Source: CAD feature listing. Evaluate the final solid. Frame: model axes, mm. A direction names the side the tool comes from. Round coordinates to 2 decimals unless told otherwise and drop trailing zeros. Write each loop counter-clockwise with the first axis right and the second up, starting at its lowest first coordinate (ties: lowest second). Pieces come first, ordered by that corner, then holes. Notation, with made-up numbers: (60, -25) - (69, -25) arc R10 cw to (69, -20) - close; hole circle Ø5 at (27, 76.5). An arc over 180 degrees is marked (long way). Write item = value, one per line. Start each with the question number.
```python
from build123d import *

# Parameters (mm, degrees)
BOSS_EXTRUDE2_DEPTH   = 3
BOSS_EXTRUDE2_2_DEPTH = 3
BOSS_EXTRUDE2_3_DEPTH = 3
BOSS_EXTRUDE2_4_DEPTH = 3
BOSS_EXTRUDE2_5_DEPTH = 3
SKETCH1_3_R           = 1.495691171
SKETCH1_3_R_2         = 1.676523608
BOSS_EXTRUDE3_DEPTH   = 2.5
SKETCH4_R             = 2
CUT_EXTRUDE5_DEPTH    = 69.0734897
CHAMFER1_SIZE         = 0.05


with BuildPart() as part:
    # Sketch1 → Boss-Extrude2 (new, symmetric)
    with BuildSketch(Plane.XY):
        with BuildLine():
            Line((-27.5, 20), (27.5, 20))
            ThreePointArc((27.5, 20), (31.035533906, 18.535533906), (32.5, 15))
            Line((32.5, 15), (32.5, -15))
            ThreePointArc((32.5, -15), (31.035533906, -18.535533906), (27.5, -20))
            Line((27.5, -20), (-27.5, -20))
            ThreePointArc((-27.5, -20), (-31.035533906, -18.535533906), (-32.5, -15))
            Line((-32.5, -15), (-32.5, 15))
            ThreePointArc((-32.5, 15), (-31.035533906, 18.535533906), (-27.5, 20))
        make_face()
        with BuildLine():
            Line((-31.5, 15), (-31.5, -15))
            ThreePointArc((-31.5, -15), (-30.328427125, -17.828427125), (-27.5, -19))
            Line((-27.5, -19), (27.5, -19))
            ThreePointArc((27.5, -19), (30.328427125, -17.828427125), (31.5, -15))
            Line((31.5, -15), (31.5, 15))
            ThreePointArc((31.5, 15), (30.328427125, 17.828427125), (27.5, 19))
            Line((27.5, 19), (-27.5, 19))
            ThreePointArc((-27.5, 19), (-30.328427125, 17.828427125), (-31.5, 15))
        make_face(mode=Mode.SUBTRACT)
    extrude(amount=BOSS_EXTRUDE2_DEPTH, both=True)



with BuildPart() as body_2:
    # Sketch1 → Boss-Extrude2 2 (new, symmetric)
    with BuildSketch(Plane.XY):
        with BuildLine():
            Line((-26.014041324, 17.60613254), (-13.852089473, 10.671658719))
            ThreePointArc((-13.852089473, 10.671658719), (-12.731915609, 6.579567504), (-16.824006824, 5.45939364))
            Line((-16.824006824, 5.45939364), (-28.985958676, 12.39386746))
            ThreePointArc((-28.985958676, 12.39386746), (-30.10613254, 16.485958676), (-26.014041324, 17.60613254))
        make_face()
        with BuildLine():
            Line((-26.261701104, 17.171777116), (-14.099749252, 10.237303296))
            ThreePointArc((-14.099749252, 10.237303296), (-13.166271032, 6.827227283), (-16.576347045, 5.893749063))
            Line((-16.576347045, 5.893749063), (-28.738298896, 12.828222884))
            ThreePointArc((-28.738298896, 12.828222884), (-29.671777116, 16.238298896), (-26.261701104, 17.171777116))
        make_face(mode=Mode.SUBTRACT)
    extrude(amount=BOSS_EXTRUDE2_2_DEPTH, both=True)


with BuildPart() as body_3:
    # Sketch1 → Boss-Extrude2 3 (new, symmetric)
    with BuildSketch(Plane.XY):
        with BuildLine():
            Line((26.014041324, 17.60613254), (13.852089473, 10.671658719))
            ThreePointArc((13.852089473, 10.671658719), (12.731915609, 6.579567504), (16.824006824, 5.45939364))
            Line((16.824006824, 5.45939364), (28.985958676, 12.39386746))
            ThreePointArc((28.985958676, 12.39386746), (30.10613254, 16.485958676), (26.014041324, 17.60613254))
        make_face()
        with BuildLine():
            Line((26.261701104, 17.171777116), (14.099749252, 10.237303296))
            ThreePointArc((14.099749252, 10.237303296), (13.166271032, 6.827227283), (16.576347045, 5.893749063))
            Line((16.576347045, 5.893749063), (28.738298896, 12.828222884))
            ThreePointArc((28.738298896, 12.828222884), (29.671777116, 16.238298896), (26.261701104, 17.171777116))
        make_face(mode=Mode.SUBTRACT)
    extrude(amount=BOSS_EXTRUDE2_3_DEPTH, both=True)


with BuildPart() as body_4:
    # Sketch1 → Boss-Extrude2 4 (new, symmetric)
    with BuildSketch(Plane.XY):
        with BuildLine():
            Line((26.014041324, -17.60613254), (13.852089473, -10.671658719))
            ThreePointArc((13.852089473, -10.671658719), (12.731915609, -6.579567504), (16.824006824, -5.45939364))
            Line((16.824006824, -5.45939364), (28.985958676, -12.39386746))
            ThreePointArc((28.985958676, -12.39386746), (30.10613254, -16.485958676), (26.014041324, -17.60613254))
        make_face()
        with BuildLine():
            Line((26.261701104, -17.171777116), (14.099749252, -10.237303296))
            ThreePointArc((14.099749252, -10.237303296), (13.166271032, -6.827227283), (16.576347045, -5.893749063))
            Line((16.576347045, -5.893749063), (28.738298896, -12.828222884))
            ThreePointArc((28.738298896, -12.828222884), (29.671777116, -16.238298896), (26.261701104, -17.171777116))
        make_face(mode=Mode.SUBTRACT)
    extrude(amount=BOSS_EXTRUDE2_4_DEPTH, both=True)


with BuildPart() as body_5:
    # Sketch1 → Boss-Extrude2 5 (new, symmetric)
    with BuildSketch(Plane.XY):
        with BuildLine():
            Line((-26.014041324, -17.60613254), (-13.852089473, -10.671658719))
            ThreePointArc((-13.852089473, -10.671658719), (-12.731915609, -6.579567504), (-16.824006824, -5.45939364))
            Line((-16.824006824, -5.45939364), (-28.985958676, -12.39386746))
            ThreePointArc((-28.985958676, -12.39386746), (-30.10613254, -16.485958676), (-26.014041324, -17.60613254))
        make_face()
        with BuildLine():
            Line((-26.261701104, -17.171777116), (-14.099749252, -10.237303296))
            ThreePointArc((-14.099749252, -10.237303296), (-13.166271032, -6.827227283), (-16.576347045, -5.893749063))
            Line((-16.576347045, -5.893749063), (-28.738298896, -12.828222884))
            ThreePointArc((-28.738298896, -12.828222884), (-29.671777116, -16.238298896), (-26.261701104, -17.171777116))
        make_face(mode=Mode.SUBTRACT)
    extrude(amount=BOSS_EXTRUDE2_5_DEPTH, both=True)


with BuildPart() as part_1:
    add(part.part)

    add(body_2.part)  # Boss-Extrude3 merges body 2

    add(body_3.part)  # Boss-Extrude3 merges body 3

    add(body_4.part)  # Boss-Extrude3 merges body 4

    add(body_5.part)  # Boss-Extrude3 merges body 5
    # Sketch1_3 → Boss-Extrude3 (add, symmetric)
    with BuildSketch(Plane.XY):
        with BuildLine():
            ThreePointArc((-27.5, 19), (-30.328427125, 17.828427125), (-31.5, 15))
            Line((-31.5, 15), (-31.5, -15))
            ThreePointArc((-31.5, -15), (-30.328427125, -17.828427125), (-27.5, -19))
            Line((-27.5, -19), (27.5, -19))
            ThreePointArc((27.5, -19), (30.328427125, -17.828427125), (31.5, -15))
            Line((31.5, -15), (31.5, 15))
            ThreePointArc((31.5, 15), (30.328427125, 17.828427125), (27.5, 19))
            Line((27.5, 19), (-27.5, 19))
        make_face()
        with BuildLine():
            Line((-13.852089473, -10.671658719), (-26.014041324, -17.60613254))
            ThreePointArc((-26.014041324, -17.60613254), (-30.10613254, -16.485958676), (-28.985958676, -12.39386746))
            Line((-28.985958676, -12.39386746), (-16.824006824, -5.45939364))
            ThreePointArc((-16.824006824, -5.45939364), (-12.731915609, -6.579567504), (-13.852089473, -10.671658719))
        make_face(mode=Mode.SUBTRACT)
        with BuildLine():
            ThreePointArc((0, -17.607662989), (-6.244508299, -12.814840409), (-8.638223432, -5.315829804))
            Line((-8.638223432, -5.315829804), (-7.540721224, -4.64044383))
            ThreePointArc((-7.540721224, -4.64044383), (-4.327491025, -12.392789568), (3.48180896, -15.465011321))
            Line((3.48180896, -15.465011321), (0, -17.607662989))
        make_face(mode=Mode.SUBTRACT)
        with Locations((4.527145443, -11.53276309)):
            Circle(SKETCH1_3_R, mode=Mode.SUBTRACT)
        with BuildLine():
            ThreePointArc((28.985958676, -12.39386746), (30.10613254, -16.485958676), (26.014041324, -17.60613254))
            Line((26.014041324, -17.60613254), (13.852089473, -10.671658719))
            ThreePointArc((13.852089473, -10.671658719), (12.731915609, -6.579567504), (16.824006824, -5.45939364))
            Line((16.824006824, -5.45939364), (28.985958676, -12.39386746))
        make_face(mode=Mode.SUBTRACT)
        with Locations((1.848455798, -6.957616723)):
            Circle(SKETCH1_3_R_2, mode=Mode.SUBTRACT)
        with BuildLine():
            ThreePointArc((-28.985958676, 12.39386746), (-30.10613254, 16.485958676), (-26.014041324, 17.60613254))
            Line((-26.014041324, 17.60613254), (-13.852089473, 10.671658719))
            ThreePointArc((-13.852089473, 10.671658719), (-12.731915609, 6.579567504), (-16.824006824, 5.45939364))
            Line((-16.824006824, 5.45939364), (-28.985958676, 12.39386746))
        make_face(mode=Mode.SUBTRACT)
        with BuildLine():
            Line((-7.540721224, 4.64044383), (-8.638223432, 5.315829804))
            ThreePointArc((-8.638223432, 5.315829804), (-6.244508299, 12.814840409), (0, 17.607662989))
            Line((0, 17.607662989), (3.48180896, 15.465011321))
            ThreePointArc((3.48180896, 15.465011321), (-4.327491025, 12.392789568), (-7.540721224, 4.64044383))
        make_face(mode=Mode.SUBTRACT)
        with Locations((1.848455798, 6.957616723)):
            Circle(SKETCH1_3_R_2, mode=Mode.SUBTRACT)
        with Locations((4.527145443, 11.53276309)):
            Circle(SKETCH1_3_R, mode=Mode.SUBTRACT)
        with BuildLine():
            Line((13.852089473, 10.671658719), (26.014041324, 17.60613254))
            ThreePointArc((26.014041324, 17.60613254), (30.10613254, 16.485958676), (28.985958676, 12.39386746))
            Line((28.985958676, 12.39386746), (16.824006824, 5.45939364))
            ThreePointArc((16.824006824, 5.45939364), (12.731915609, 6.579567504), (13.852089473, 10.671658719))
        make_face(mode=Mode.SUBTRACT)
    extrude(amount=BOSS_EXTRUDE3_DEPTH, both=True)

    # Sketch4 → Cut-Extrude5 (cut, through all)
    with BuildSketch(Plane.ZY.offset(32.5)):
        with Locations(Location((0, 0, 0), (0, 0, 270))):
            Circle(SKETCH4_R)
    extrude(amount=-CUT_EXTRUDE5_DEPTH, mode=Mode.SUBTRACT)

    # Chamfer1
    chamfer1_edges = [part_1.edges().sort_by_distance(p)[0] for p in [
        (32.5, 2, 0),
        (-32.5, 2, 0),
    ]]
    chamfer(chamfer1_edges, length=CHAMFER1_SIZE)


solid = part_1.part
```
(1) Ray query, L1, parallel to Z at x = -5, y = 0; L2, parallel to X at y = 11, z = 1.8; L3, parallel to Y at x = 26.5, z = -0.6. Return the intervals inside material, ascending. Write a range as from..to.
(2) Section B-B (z = 0). Count the separate pieces of the cut face and the enclosed holes in it, plus the area to 3 significant figures.
(3) Reachability of faces 1 (the flat face through (-20.266, 13.753, 0.042)), 2 (the flat face through (-23.5, -9.6, -3)), 3 (the cylindrical face through (-30.359, -17.797, 2.754)), 4 (the cylindrical face through (-12.7, -6.64, -2.75)) from +Z, -Z, +X, -X, +Y, -Y: full face, straight path, thin tool, end or side. Return the list, or none.
(4) Section A-A (y = 0). Return the cut outline in (x, z).
(5) Pull-direction query (X, two-part tool) for faces 5 (the flat face through (19.4, 13.5, -3)), 6 (the flat face through (-20.266, -13.753, 0.042)), 7 (the cylindrical face through (-31, -18.57, 0.04)); classes: +X half, -X half, draft (parallel to the pull), parting line (faces both ways), or undercut.
(6) Contact query for flat-ended pins moving along their axis: P1, Ø2.5, axis at y = 0, z = 0, coming from the -X side; P2, Ø4, axis at x = -9.5, y = 1, coming from the +Z side; P3, Ø10, axis at x = 18, y = 16, coming from the +Z side; P4, Ø2, axis at x = 14, y = -3, coming from the -Z side. Output: stop coordinate, or through.
Solution:
q1.L1 = -2.5..-2, 2..2.5
q1.L2 = -32.5..-25.53, -15.44..-7.31, -5.52..3.13, 5.92..15.44, 25.53..32.5
q1.L3 = -20..-17.29, -11.55..-1.91, 1.91..11.55, 17.29..20
q2.separate_pieces = 2
q2.enclosed_holes = 10
q2.area = 1,870 mm^2
q3.face_1 = +Z, -Z
q3.face_2 = -Z, +X, -X, +Y, -Y
q3.face_3 = +Z
q3.face_4 = -Z
q4.outline = (-32.5, -3) - (-31.5, -3) - (-31.5, -2.5) - (31.5, -2.5) - (31.5, -3) - (32.5, -3) - (32.5, -2.05) - (32.45, -2) - (-32.45, -2) - (-32.5, -2.05) - close; (-32.5, 2.05) - (-32.45, 2) - (32.45, 2) - (32.5, 2.05) - (32.5, 3) - (31.5, 3) - (31.5, 2.5) - (-31.5, 2.5) - (-31.5, 3) - (-32.5, 3) - close
q5.face_5 = draft
q5.face_6 = undercut
q5.face_7 = -X half
q6.P1 = through
q6.P2 = 2.5
q6.P3 = 3
q6.P4 = -2.5
